Here's how the part is built. I have some questions about the finished solid (model axes, mm). A direction names the side the tool comes from. Give positions to 0.01 mm unless a question says otherwise; leave off trailing zeros. Write each loop counter-clockwise with the first axis right and the second up, starting at its lowest first coordinate (ties: lowest second). Pieces come first, ordered by that corner, then holes. Notation, with made-up numbers: (63.5, 27) -> (74.5, 27) arc R30 cw to (74.5, 66) -> close; hole circle Ø5 at (39.25, 68). An arc over 180 degrees is marked (long way). Put each result on its own line as item: value. Start each with the question number.
from build123d import *

# Parameters (mm, degrees)
PAD048_DEPTH    = 7
SKETCH145_R     = 5
PAD052_DEPTH    = 5
SKETCH146_R     = 2.3
POCKET042_DEPTH = 5.5


with BuildPart() as part:
    # Sketch134 → Pad048 (new body)
    with BuildSketch(Plane.XY):
        with BuildLine():
            Line((28.913665, 126), (78.342597, 126))
            ThreePointArc((78.342597, 110), (86.342597, 118), (78.342597, 126))
            Line((28.913665, 110), (78.342597, 110))
            ThreePointArc((8, 89.086335), (21.213203, 96.786797), (28.913665, 110))
            Line((8, 89.086335), (8, 39.657403))
            ThreePointArc((-8, 39.657403), (0, 31.657429), (8, 39.657403))
            Line((-8, 89.086335), (-8, 39.657403))
            ThreePointArc((-28.913665, 110), (-21.213203, 96.786797), (-8, 89.086335))
            Line((-28.913665, 110), (-78.342597, 110))
            ThreePointArc((-78.342597, 126), (-86.342605, 118), (-78.342597, 110))
            Line((-28.913665, 126), (-78.342597, 126))
            ThreePointArc((-8, 146.913665), (-21.213203, 139.213203), (-28.913665, 126))
            Line((-8, 146.913665), (-8, 196.342597))
            ThreePointArc((8, 196.342597), (0, 204.342636), (-8, 196.342597))
            Line((8, 196.342597), (8, 146.913665))
            ThreePointArc((28.913665, 126), (21.213203, 139.213203), (8, 146.913665))
        make_face()
    extrude(amount=PAD048_DEPTH)

    # Sketch145 → Pad052 (join)
    with BuildSketch(Plane(origin=(0, 0, 0), x_dir=(1, 0, 0), z_dir=(0, 0, -1))):
        with Locations((0, -38.25)):
            Circle(SKETCH145_R)
        with Locations((0, -197.75)):
            Circle(SKETCH145_R)
        with Locations((-79.75, -118)):
            Circle(SKETCH145_R)
        with Locations((79.75, -118)):
            Circle(SKETCH145_R)
    extrude(amount=PAD052_DEPTH)

    # Sketch146 (on Face5 of Pad052) → Pocket042 (cut)
    with BuildSketch(Plane.XY.offset(7)):
        with Locations((-10.606602, 128.606602)):
            Circle(SKETCH146_R)
        with Locations((10.606602, 128.606602)):
            Circle(SKETCH146_R)
        with Locations((10.606602, 107.393398)):
            Circle(SKETCH146_R)
        with Locations((-10.606602, 107.393398)):
            Circle(SKETCH146_R)
    extrude(amount=-POCKET042_DEPTH, mode=Mode.SUBTRACT)


with BuildPart() as part_1:
    # Body021 placement: moved
    add(part.part.moved(Location((0, 0, 35))))


solid = part_1.part
1) I want a section at D-D, the plane y = 155. Write out the boundary of the cut face in (x, z), and give its area (3 significant figures).
2) I want a section at B-B, the plane y = 118. Write out the boundary of the cut face in (x, z).
3) I'm going to push flat-ended pins straight in: pin 1 Ø1.5 at (y, z) = (120.5, 33.5) entering from +X; pin 2 Ø5.5 at (x, z) = (-58, 40) entering from -Y; pin 3 Ø2 at (x, z) = (46.5, 39.5) entering from +Y; pin 4 Ø5 at (x, y) = (11, 106.5) entering from +Z. Where does each tip first touch, or does it pass through?
4) I want a section at A-A, the plane x = 0. Write out the boundary of the cut face in (y, z), and give its area (3 significant figures).
5) I need wall thicknesses on probe 1 along Y at (x, z) = (-55.5, 37.5); probe 2 along X at (y, z) = (184, 37.5); probe 3 along Y at (x, z) = (-4.5, 32.25). Which ranges of each line are inside material? Lowest first, please.
6) I want a section at C-C, the plane x = -32.5. Write out the boundary of the cut face in (y, z), and give its area (3 significant figures).
7) Thinking about a two-plate mould opening in X: for faces 1 (the flat face through (0, 38, 30)), 2 (the cylindrical face through (-86.34, 118.18, 38.45)), 3 (the flat face through (11, 129, 36.5)), which applies, released by +X, released by -X, zero draft, split by the parting line, or undercut?
8) Which directions (+Z, -Z, +X, -X, +Y, -Y) give clear straight access to the entire face, cutting with the end or side of a thin tool? Please do faces 4 (the flat face through (-11, 107, 36.5)), 5 (the flat face through (8, 65, 38)), 6 (the flat face through (0, 118, 35)), 7 (the flat face through (8, 172, 38)).
Established:
1. outline: (-8, 35) -> (8, 35) -> (8, 42) -> (-8, 42) -> close
1. area: 112 mm2
2. outline: (-86.34, 35) -> (-84.75, 35) -> (-84.75, 30) -> (-74.75, 30) -> (-74.75, 35) -> (74.75, 35) -> (74.75, 30) -> (84.75, 30) -> (84.75, 35) -> (86.34, 35) -> (86.34, 42) -> (-86.34, 42) -> close
3. pin 1: stops at x = 84.43
3. pin 2: stops at y = 110
3. pin 3: stops at y = 126
3. pin 4: stops at z = 42
4. outline: (31.66, 35) -> (33.25, 35) -> (33.25, 30) -> (43.25, 30) -> (43.25, 35) -> (192.75, 35) -> (192.75, 30) -> (202.75, 30) -> (202.75, 35) -> (204.34, 35) -> (204.34, 42) -> (31.66, 42) -> close
4. area: 1,310 mm2
5. probe 1: y = 110 to 126
5. probe 2: x = -8 to 8
5. probe 3: y = 36.07 to 40.43, 195.57 to 199.93
6. outline: (110, 35) -> (126, 35) -> (126, 42) -> (110, 42) -> close
6. area: 112 mm2
7. face 1: zero draft
7. face 2: released by -X
7. face 3: undercut
8. face 4: +Z
8. face 5: +Z, -Z, +X, -Y
8. face 6: -Z
8. face 7: +Z, -Z, +X, +Y
